Work out the finished part from the listing and answer in its coordinate system (mm). Face numbers are marked on the shaded views. A direction names the side the tool comes from. Give positions to 0.01 mm unless a question says otherwise; leave off trailing zeros. Write each loop counter-clockwise with the first axis right and the second up, starting at its lowest first coordinate (ties: lowest second). Pieces come first, ordered by that corner, then holes. Notation, with made-up numbers: (69.25, 46.5) - (99.25, 46.5) arc R3 ccw to (99.25, 50.5) - close; hole circle Ø2 at (-33, -27). An arc over 180 degrees is marked (long way). Write item = value, one per line.
from build123d import *

# Parameters (mm, degrees)
BOSS_EXTRUDE2_DEPTH = 10


with BuildPart() as part:
    # Sketch2 → Boss-Extrude2 (new body)
    with BuildSketch(Plane.XY):
        with BuildLine():
            Line((0, 19.454800467), (0, 5))
            Line((0, 5), (2.886751346, 5))
            Line((2.886751346, 5), (4.330127019, 2.5))
            Line((4.330127019, 2.5), (13.002406473, 2.5))
            Line((13.002406473, 2.5), (13.002406473, 7.5))
            Line((13.002406473, 7.5), (11.039564591, 7.5))
            Line((11.039564591, 7.5), (11.039564591, 10.2))
            Line((11.039564591, 10.2), (13.002406473, 10.2))
            Line((13.002406473, 10.2), (13.002406473, 13.7))
            Line((13.002406473, 13.7), (16.202406473, 13.7))
            Line((16.202406473, 13.7), (16.202406473, 10.2))
            Line((16.202406473, 10.2), (18.165248356, 10.2))
            Line((18.165248356, 10.2), (18.165248356, 7.5))
            Line((18.165248356, 7.5), (16.202406473, 7.5))
            Line((16.202406473, 7.5), (16.202406473, 2.5))
            Line((16.202406473, 2.5), (24.874685928, 2.5))
            ThreePointArc((24.874685928, 2.5), (21.987632849, 11.89722664), (15.700660457, 19.454800467))
            Line((15.700660457, 19.454800467), (0, 19.454800467))
        make_face()
        with BuildLine():
            Line((-13.002406473, 2.5), (-4.330127019, 2.5))
            Line((-4.330127019, 2.5), (-2.886751346, 5))
            Line((-2.886751346, 5), (0, 5))
            Line((0, 5), (0, 19.454800467))
            Line((0, 19.454800467), (-15.700660457, 19.454800467))
            ThreePointArc((-15.700660457, 19.454800467), (-21.987632849, 11.89722664), (-24.874685928, 2.5))
            Line((-24.874685928, 2.5), (-16.202406473, 2.5))
            Line((-16.202406473, 2.5), (-16.202406473, 7.5))
            Line((-16.202406473, 7.5), (-18.165248356, 7.5))
            Line((-18.165248356, 7.5), (-18.165248356, 10.2))
            Line((-18.165248356, 10.2), (-16.202406473, 10.2))
            Line((-16.202406473, 10.2), (-16.202406473, 13.7))
            Line((-16.202406473, 13.7), (-13.002406473, 13.7))
            Line((-13.002406473, 13.7), (-13.002406473, 10.2))
            Line((-13.002406473, 10.2), (-11.039564591, 10.2))
            Line((-11.039564591, 10.2), (-11.039564591, 7.5))
            Line((-11.039564591, 7.5), (-13.002406473, 7.5))
            Line((-13.002406473, 7.5), (-13.002406473, 2.5))
        make_face()
    extrude(amount=BOSS_EXTRUDE2_DEPTH)


solid = part.part
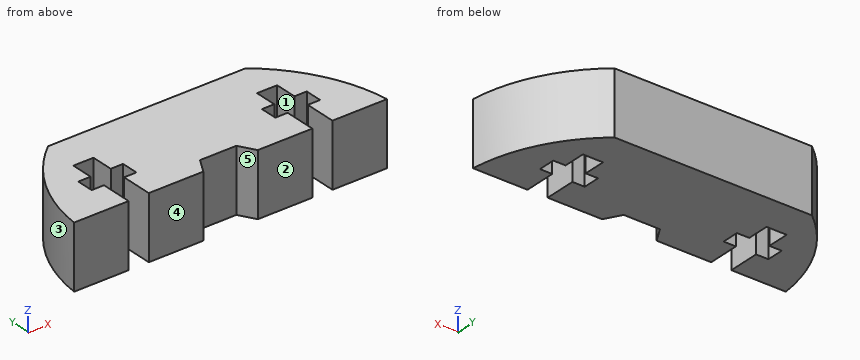
1. Given pin 1 (4.5 mm diameter, centred on x = -1, z = 4, fed in from -Y); pin 2 (2.5 mm diameter, centred on y = 4.5, z = 5.5, fed in from +X); pin 3 (2 mm diameter, centred on x = -17, z = 5.5, fed in from +Y); pin 4 (1.5 mm diameter, centred on x = -14.5, y = 12, fed in from +Z), each flat-ended and moving along its own axis, determine where each tip first touches the part or whether it passes through.
Solution:
pin_1 = 4.37
pin_2 = 24.79
pin_3 = 19.21
pin_4 = through
2. Find section B-B, the plane y = 10.75. Give the vertices of the cut face in (x, z), then the cut area to 3 significant figures.
Solution:
outline = (-22.57, 0) - (-16.2, 0) - (-16.2, 10) - (-22.57, 10) - close; (-13, 0) - (13, 0) - (13, 10) - (-13, 10) - close; (16.2, 0) - (22.57, 0) - (22.57, 10) - (16.2, 10) - close
area = 387 mm^2
3. Straight lines are drawn through the part: line 1 (X direction, y = 3.75, z = 3.75); line 2 (X direction, y = 12.75, z = 7); line 3 (X direction, y = 8.5, z = 1.5). For each, find the intervals that lie inside material, in ascending order.
Solution:
line_1 = -24.72 to -16.2, -13 to -3.61, 3.61 to 13, 16.2 to 24.72
line_2 = -21.5 to -16.2, -13 to 13, 16.2 to 21.5
line_3 = -23.51 to -18.17, -11.04 to 11.04, 18.17 to 23.51
4. For a pull along X with two mould halves and no side action, classify the marked faces 1, 2 and 3 as pulls with the +X half, pulls with the -X half, needs draft (parallel to the pull), parting line crosses it, or undercut.
Solution:
face_1 = undercut
face_2 = needs draft
face_3 = pulls with the -X half
5. Find section A-A, the plane x = 12. Give the vertices of the cut face in (y, z), then the cut area to 3 significant figures.
Solution:
outline = (2.5, 0) - (7.5, 0) - (7.5, 10) - (2.5, 10) - close; (10.2, 0) - (19.45, 0) - (19.45, 10) - (10.2, 10) - close
area = 143 mm^2
6. Find section D-D, the plane x = 2. Give the vertices of the cut face in (y, z), then the cut area to 3 significant figures.
Solution:
outline = (5, 0) - (19.45, 0) - (19.45, 10) - (5, 10) - close
area = 145 mm^2
7. A tool of negligible diameter and unlimited length cuts with its end or side. For the marked faces 4 and 5, from which of +Z, -Z, +X, -X, +Y, -Y can it reach the whole face along a straight path? Write none if from no direction.
Solution:
face_4 = +Z, -Z, +X, -X, -Y
face_5 = +Z, -Z, -Y
